Verification items for the finished model (mm, model axes). A direction names the side the tool comes from. Coordinates: 2 decimals unless noted, no trailing zeros. Loops run counter-clockwise (first coordinate to the right, second up) from the corner with the lowest first, then second, coordinate; pieces in that order, holes last. Notation, with made-up numbers: M 31,-5.5 L 83,-5.5 A18 cw 83,25.5 Z; hole C 71,-32.5 d11. An arc over 180 degrees is marked long. Write item = value, one per line. Start each with the question number.
Autodesk Inventor part; units mm, degrees
ref_plane "YZ Plane" through (0, 0, 0) normal (1, 0, 0) x (0, 1, 0)
ref_plane "XZ Plane" through (0, 0, 0) normal (0, 1, 0) x (-1, 0, 0)
ref_plane "XY Plane" through (0, 0, 0) normal (0, 0, 1) x (1, 0, 0)
sketch "Sketch1" plane through (0, 0, 0) normal (0, 1, 0) x (-1, 0, 0)
  line L0 (0, 0) -> (20, 0)
  line L1 (20, 0) -> (20, -3)
  line L2 (20, -3) -> (0, -3)
  line L3 (0, -3) -> (0, 0)
  line L4 (0, 0) -> (3, 0)
  line L5 (3, 0) -> (3, -20)
  line L6 (3, -20) -> (0, -20)
  line L7 (0, -20) -> (0, 0)
  dimension "d0" = 3
  dimension "d1" = 3
  dimension "d2" = 20
  dimension "d3" = 20
extrude "Extrusion1" add sketch "Sketch1" along normal blind 40
fillet "Fillet1" radius 2 1 edges at (-3, 20, -3)
fillet "Fillet2" radius 5 1 edges at (0, 20, 0)
sketch "Sketch2" plane through (-3, 0, -20) normal (-1, 0, 0) x (0, 0, 1)
  line L0 (0, 40) -> (15, 40)
  line L1 (0, 0) -> (15, 0)
  line L2 (0, 0) -> (0, 40)
  point P0 (20, 0)
  point P1 (7.5, 32.5)
  point P2 (7.5, 7.5)
  dimension "d8" = 7.5
  dimension "d9" = 7.5
  dimension "d10" = 25
  dimension "d11" = 7.5
hole "Hole1" at (-3, 32.5, -12.5) at (-3, 7.5, -12.5) direction (1, 0, 0) diameter 4.5 end through all
sketch "Sketch3" plane through (-20, 0, -3) normal (0, 0, -1) x (-1, 0, 0)
  line L0 (-15, 40) -> (0, 40)
  line L1 (-15, 0) -> (0, 0)
  line L2 (0, 0) -> (0, 40)
  point P0 (-20, 0)
  point P1 (-7.5, 32.5)
  point P2 (-7.5, 7.5)
  dimension "d19" = 7.5
  dimension "d20" = 7.5
  dimension "d21" = 7.5
hole "Hole2" at (-12.5, 32.5, -3) at (-12.5, 7.5, -3) direction (0, 0, 1) diameter 4.5 end through all
equation "\"d1\" = d0"
equation "\"d3\" = d2"
properties part number "Timing_Angle Bracket" material "Aluminum 6061"
Q1. Mould release check, pull along Z, two halves, no side actions. Record for faces 1 (the face through (-1.48, 5.98, -14.16)), 2 (the face through (-2, 20, -20)), 3 (the face through (-2.5, 40, -7)): +Z half, -Z half, draft (parallel to the pull), parting line (faces both ways), or undercut.
Q2. Sectioned sample at B-B on z = -12.5. Record the cut outline in (x, y).
Q3. Sectioned sample at C-C on x = -11. Record the cut outline in (y, z), plus the area to 3 significant figures.
Q4. Gauge pin test, flat ends, axial feed: pin 1 (4.5 mm diameter, centred on y = 16.5, z = -10, fed in from -X); pin 2 (2 mm diameter, centred on x = -8.5, z = -5, fed in from -Y); pin 3 (2 mm diameter, centred on x = -4.5, y = 28.5, fed in from -Z). Record the tip position at first contact, or that the pin passes through.
Q5. Sectioned sample at A-A on y = 7.5. Record the cut outline in (x, z).
Q6. Set-up check for faces 4 (the face through (-13, 20, -3)), 5 (the face through (0, 20, -13)): record each of +Z, -Z, +X, -X, +Y, -Y from which the full face is reachable in a straight line by a thin tool's end or side.
Q7. Scan lines: L1, parallel to Y at x = -11.75, z = -2.75; L2, parallel to Y at x = -2.2, z = -12.5; L3, parallel to Z at x = -10, y = 17. Record each from-to range of solid material in increasing order. Write a range as [from, to].
Q8. Sectioned sample at D-D on y = 19. Record the cut outline in (x, z).
Solutions:
q1.face_1 = undercut
q1.face_2 = -Z half
q1.face_3 = draft
q2.outline = M -3,0 L 0,0 L 0,5.25 L -3,5.25 Z; M -3,9.75 L 0,9.75 L 0,30.25 L -3,30.25 Z; M -3,34.75 L 0,34.75 L 0,40 L -3,40 Z
q3.outline = M 0,-3 L 5.82,-3 L 5.82,0 L 0,0 Z; M 9.18,-3 L 30.82,-3 L 30.82,0 L 9.18,0 Z; M 34.18,-3 L 40,-3 L 40,0 L 34.18,0 Z
q3.area = 99.9 mm²
q4.pin_1 = -3
q4.pin_2 = through
q4.pin_3 = -3.68
q5.outline = M -20,-3 L -14.75,-3 L -14.75,0 L -20,0 Z; M -10.25,-3 L -5,-3 A2 cw -3,-5 L -3,-10.25 L 0,-10.25 L 0,-5 A5 ccw -5,0 L -10.25,0 Z; M -3,-20 L 0,-20 L 0,-14.75 L -3,-14.75 Z
q6.face_4 = -Z, -X, +Y, -Y
q6.face_5 = +Z, -Z, +X, +Y, -Y
q7.L1 = [0, 5.38], [9.62, 30.38], [34.62, 40]
q7.L2 = [0, 5.25], [9.75, 30.25], [34.75, 40]
q7.L3 = [-3, 0]
q8.outline = M -20,-3 L -5,-3 A2 cw -3,-5 L -3,-20 L 0,-20 L 0,-5 A5 ccw -5,0 L -20,0 Z
